from build123d import *

# Parameters (mm, degrees)
SKETCH1_R           = 17.5
BOSS_EXTRUDE1_DEPTH = 5
SKETCH2_R           = 17.5
SKETCH2_R_2         = 15
BOSS_EXTRUDE2_DEPTH = 15
SKETCH3_R           = 7.5
CUT_EXTRUDE1_DEPTH  = 21
CHAMFER1_SIZE       = 2


with BuildPart() as part:
    # Sketch1 → Boss-Extrude1 (new body)
    with BuildSketch(Plane.XY):
        Circle(SKETCH1_R)
    extrude(amount=BOSS_EXTRUDE1_DEPTH)

    # Sketch2 → Boss-Extrude2 (add)
    with BuildSketch(Plane.XY.offset(5)):
        Circle(SKETCH2_R)
        Circle(SKETCH2_R_2, mode=Mode.SUBTRACT)
    extrude(amount=BOSS_EXTRUDE2_DEPTH)

    # Sketch3 → Cut-Extrude1 (cut, through all)
    with BuildSketch(Plane(origin=(0, 0, 0), x_dir=(-1, 0, 0), z_dir=(0, 0, -1))):
        Circle(SKETCH3_R)
    extrude(amount=-CUT_EXTRUDE1_DEPTH, mode=Mode.SUBTRACT)

    # Chamfer1
    chamfer1_edges = [part.edges().sort_by_distance(p)[0] for p in [
        (-17.5, 0, 0),
    ]]
    chamfer(chamfer1_edges, length=CHAMFER1_SIZE)


solid = part.part
Work out the finished part from the listing and answer in its coordinate system (mm). Round coordinates to 2 decimals unless told otherwise and drop trailing zeros. Write each loop counter-clockwise with the first axis right and the second up, starting at its lowest first coordinate (ties: lowest second). Pieces come first, ordered by that corner, then holes.
1) Straight lines are drawn through the part: line 1 (Y direction, x = 0, z = 4); line 2 (Y direction, x = 0, z = 11.25); line 3 (X direction, y = -0.5, z = 18.5). For each, find the intervals that lie inside material, in ascending order.
2) A cutting plane is placed at A-A (y = 0). Give the vertices of the cut face in (x, z).
3) The mould has two halves that part along X. Classify faces 1 (the cylindrical face through (-13.887, -10.648, 10.874)), 2 (the flat face through (-4, -7, 0)), 3 (the cylindrical face through (-14.985, 0.66, 12.395)), 4 (the flat face through (-4, 7, 5)): pulls with the +X half, pulls with the -X half, needs draft (parallel to the pull), parting line crosses it, or undercut.
4) Given pin 1 Ø10 at (x, z) = (-12, 10.5) entering from -Y; pin 2 Ø4 at (x, z) = (5.5, 4.5) entering from +Y; pin 3 Ø9 at (x, y) = (1, 6.5) entering from +Z, each flat-ended and moving along its own axis, determine where each tip first touches the part or whether it passes through.
5) A cutting plane is placed at C-C (z = 8.25). Give the vertices of the cut face in (x, y).
Completed:
1. line 1: y = -17.5 to -7.5, 7.5 to 17.5
1. line 2: y = -17.5 to -15, 15 to 17.5
1. line 3: x = -17.49 to -14.99, 14.99 to 17.49
2. outline: (-17.5, 2) - (-15.5, 0) - (-7.5, 0) - (-7.5, 5) - (-15, 5) - (-15, 20) - (-17.5, 20) - close; (7.5, 0) - (15.5, 0) - (17.5, 2) - (17.5, 20) - (15, 20) - (15, 5) - (7.5, 5) - close
3. face 1: parting line crosses it
3. face 2: needs draft
3. face 3: undercut
3. face 4: undercut
4. pin 1: stops at y = -16.04
4. pin 2: stops at y = 17.15
4. pin 3: stops at z = 5
5. outline: circle Ø35 at (0, 0); hole circle Ø30 at (0, 0)
